Autodesk Inventor part; units mm, degrees
ref_plane "Work Plane1" through (30, 0, 0) normal (1, 0, 0) x (0, 1, 0)
ref_plane "XZ Plane" through (0, 0, 0) normal (0, 1, 0) x (-1, 0, 0)
ref_plane "XY Plane" through (0, 0, 0) normal (0, 0, 1) x (1, 0, 0)
sketch "Sketch1" plane through (0, 0, 0) normal (1, 0, 0) x (0, 1, 0)
  arc A0 (7.4985, -0.1486) -> (-3.2805, 6.7445) centre (0, 0) ccw
  line L0 (0, 0) -> (-1.75, 0)
  line L1 (-1.75, 0) -> (-1.75, -0.1486)
  line L2 (-1.75, -4.1458) -> (-0.74, -4.1458) construction
  line L3 (-3.2805, 6.7445) -> (-3.0298, 6.3103)
  line L4 (-3.2805, 6.7445) -> (-2.7791, 6.7445) construction
  line L5 (6.9984, -0.1486) -> (16.9984, -0.1486)
  line L6 (16.9984, -0.1486) -> (16.9984, 2.8514)
  line L7 (16.9984, 2.8514) -> (1.2284, 7.4544)
  arc A1 (6.9984, -0.1486) -> (-3.0298, 6.3103) centre (0, 0) ccw
  point P0 (2.1014, 7.1996)
  dimension "d1" = 15
  dimension "d2" = 1.75
  dimension "d4" = 60
  dimension "d5" = 10
  dimension "d6" = 3
  dimension "d8" = 7
revolve "Revolution1" add sketch "Sketch1" angle 360 about axis through (0, 6.9984, -0.1486) along (0, 1, 0)
ref_plane "Work Plane1" through (30, 0, 0) normal (1, 0, 0) x (0, 1, 0)
sketch "Sketch2" plane through (30, 0, 0) normal (1, 0, 0) x (0, 1, 0)
  line L0 (16.9984, -3.1486) -> (16.9984, 2.8514)
  line L1 (14.9984, 2.8514) -> (6.9984, 2.8514)
  line L2 (14.9984, -3.1486) -> (6.9984, -3.1486)
  line L3 (16.9984, 0.8514) -> (16.9984, -1.1486)
  arc A0 (16.9984, 0.8514) -> (14.9984, 2.8514) centre (14.9984, 0.8514) ccw
  arc A1 (14.9984, -3.1486) -> (16.9984, -1.1486) centre (14.9984, -1.1486) ccw
  line L4 (6.9984, 2.8514) -> (6.9984, 7.8514)
  line L5 (6.9984, 7.8514) -> (1.9984, 7.8514)
  line L6 (1.9984, 7.8514) -> (1.9984, -8.1486)
  line L7 (2.1014, -7.4967) -> (2.1014, 7.1996)
  line L8 (1.9984, 7.8514) -> (17.9984, 7.8514) construction
  line L9 (1.9984, -8.1486) -> (6.9984, -8.1486)
  line L10 (6.9984, -8.1486) -> (6.9984, -3.1486)
  point P0 (0, 0)
  dimension "d10" = 10
  dimension "d11" = 10
  dimension "d12" = 2
  dimension "d13" = 5
  dimension "d14" = 5
  dimension "d15" = 16
  dimension "d16" = 90
  dimension "d17" = 5
extrude "Extrusion1" add sketch "Sketch2" against normal blind 3
sketch "Sketch3" plane through (27, 0, 0) normal (-1, 0, 0) x (0, 0, 1)
  line L0 (0.8514, 16.9984) -> (-1.1486, 16.9984)
  line L1 (-0.1486, 16.9984) -> (-0.1486, 8.9984)
  line L2 (-0.1486, 8.9984) -> (-3.1486, 8.9984)
  line L3 (-3.1486, 14.9984) -> (-3.1486, 6.9984)
  line L4 (-0.1486, 8.9984) -> (2.8514, 8.9984)
  line L5 (2.8514, 6.9984) -> (2.8514, 14.9984)
  arc A0 (2.8514, 14.9984) -> (0.8514, 16.9984) centre (0.8514, 14.9984) ccw
  arc A1 (-1.1486, 16.9984) -> (-3.1486, 14.9984) centre (-1.1486, 14.9984) ccw
  point P0 (0, 0)
  dimension "d20" = 8
extrude "Extrusion2" add sketch "Sketch3" along normal up to surface
fillet "Fillet1" radius 2 4 edges at (28.5, 1.9984, -8.1486) (28.5, 6.9984, -8.1486) (28.5, 1.9984, 7.8514) (28.5, 6.9984, 7.8514)
sketch "Sketch4" plane through (30, 0, 0) normal (1, 0, 0) x (0, 0, -1)
  line L0 (8.1486, 4.9984) -> (8.1486, 3.9984)
  line L1 (8.1486, 4.4984) -> (5.6486, 4.4984)
  circle A0 centre (5.6486, 4.4984) radius 1
  line L2 (-7.8514, 4.9984) -> (-7.8514, 3.9984)
  line L3 (-7.8514, 4.4984) -> (-5.3514, 4.4984)
  circle A1 centre (-5.3514, 4.4984) radius 1
  point P0 (0, 0)
  dimension "d24" = 2.5
  dimension "d25" = 2
  dimension "d26" = 2.5
  dimension "d27" = 2
extrude "Extrusion3" cut sketch "Sketch4" against normal up to surface (3 mm away)
sketch "Sketch5" plane through (27, 0, 0) normal (-1, 0, 0) x (0, 0, 1)
  circle A0 centre (5.3514, 4.4984) radius 1
  circle A1 centre (-5.6486, 4.4984) radius 1
  circle A2 centre (-5.6486, 4.4984) radius 1.7
  circle A3 centre (5.3514, 4.4984) radius 1.7
  point P0 (0, 0)
  dimension "d30" = 3.4
  dimension "d31" = 3.4
extrude "Extrusion4" cut sketch "Sketch5" against normal blind 1.5
equation "\"d21\" = d20"
properties part number "BallFemale"
Can you work these out from the model? Positions are in its coordinate system, mm. A direction names the side the tool comes from. Give positions to 0.01 mm unless a question says otherwise; leave off trailing zeros. Order: outer loops, then holes, each group sorted by start corner. A loop starts at its lowest first (then second) coordinate and runs counter-clockwise, first axis right, second up. Notation, with made-up numbers: M 81.5,61 L 91.5,61 A19 cw 91.5,95 Z; hole C -18.5,47 d1. An arc over 180 degrees is marked long. Write item = value, one per line. Start each with the question number.
Q1. We'd pull the mould along Z, two halves only. Please class faces 1 (the flat face through (16, 12, 2.851)), 2 (the cylindrical face through (27.7, 3.8, -4.1)), 3 (the cylindrical face through (28.479, 6.428, -7.547)): pulls with the +Z half, pulls with the -Z half, needs draft (parallel to the pull), parting line crosses it, or undercut.
Q2. For faces 4 (the flat face through (29, 1.998, 0)), 5 (the flat face through (29, 6.998, -5)), 6 (the flat face through (27, 5, 0)), 7 (the flat face through (28.5, 3, -6)), 8 (the cylindrical face through (28.48, 2.6, -7.58)), which set-ups out of +Z, -Z, +X, -X, +Y, -Y let a thin tool reach every point of the face, with its end or its side?
Q3. Suppose I cut it at A-A (y = 8.5). Write out the boundary of the cut face in (x, z).
Q4. Will these pins go through, and if not, where does the flat tip stop? pin 1 Ø2.5 at (y, z) = (4.5, 5.35) entering from -X; pin 2 Ø5.5 at (y, z) = (4.5, -5.65) entering from -X; pin 3 Ø1.8 at (y, z) = (4.5, 5.35) entering from +X.
Q5. Suppose I cut it at D-D (y = 13.5). Write out the boundary of the cut face in (x, z).
Q6. Suppose I cut it at C-C (z = 5). Count the separate pieces of the cut face and the enclosed holes in it, plus the area to 3 significant figures.
Q7. I need wall thicknesses on probe 1 along X at (y, z) = (4, 4); probe 2 along Z at (x, y) = (19.5, 10.75); probe 3 along Z at (x, y) = (-2.5, -0.75). Which ranges of each line are inside material? Lowest first, please. Write a range as [from, to].
Q8. Suppose I cut it at B-B (x = 25). Write out the boundary of the cut face in (y, z).
Check result:
q1.face_1 = pulls with the +Z half
q1.face_2 = undercut
q1.face_3 = pulls with the -Z half
q2.face_4 = +Z, -Z, +X, -Y
q2.face_5 = -Z, +X, +Y
q2.face_6 = +Z, -Z, -Y
q2.face_7 = none
q2.face_8 = -Z, +X, -Y
q3.outline = C 0,-0.15 d10.96; M 27,-3.15 L 30,-3.15 L 30,2.85 L 27,2.85 Z
q4.pin_1 = -5.22
q4.pin_2 = -6.32
q4.pin_3 = 4.87
q5.outline = M 2.68,-3.15 L 30,-3.15 L 30,2.85 L 2.68,2.85 A4.02 ccw long Z
q6.separate_pieces = 3
q6.enclosed_holes = 0
q6.area = 47.7 mm2
q7.probe_1 = [-5.38, -4.19], [4.19, 5.38], [28.5, 30]
q7.probe_2 = [-3.15, 2.85]
q7.probe_3 = [-7.34, -6.8], [6.51, 7.04]
q8.outline = M 9,-3.15 L 15,-3.15 A2 ccw 17,-1.15 L 17,0.85 A2 ccw 15,2.85 L 9,2.85 Z
